Here's how the part is built. I have some questions about the finished solid (model axes, mm). Coordinates: 2 decimals unless noted, no trailing zeros. Write each loop counter-clockwise with the first axis right and the second up, starting at its lowest first coordinate (ties: lowest second). Pieces come first, ordered by that corner, then holes.
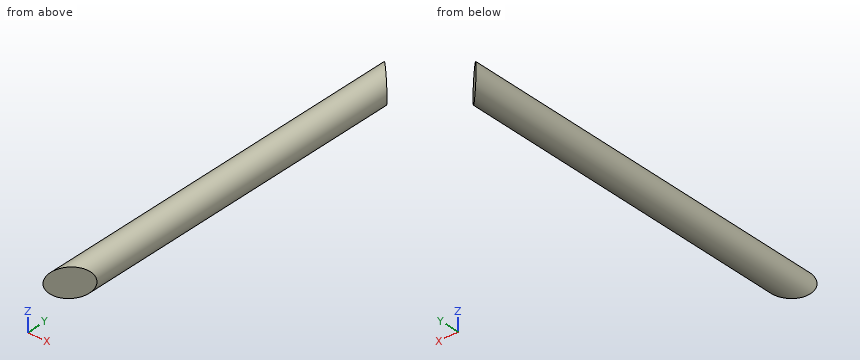
```python
from build123d import *

# Parameters (mm, degrees)
SKETCH1_R               = 31.75
BOSS_EXTRUDE1_DEPTH     = 723.9
SKETCH4_R               = 31.75
BOSS_EXTRUDE2_DEPTH     = 63.5
SKETCH5_R               = 31.75
BOSS_EXTRUDE3_DEPTH     = 63.5
CUT_EXTRUDE2_DEPTH      = 63.5
CUT_EXTRUDE2_DEPTH_BACK = 63.5


with BuildPart() as part:
    # Sketch1 → Boss-Extrude1 (new body)
    with BuildSketch(Plane(origin=(0, 0, 0), x_dir=(1, 0, 0), z_dir=(0, 1, 0))):
        Circle(SKETCH1_R)
    extrude(amount=BOSS_EXTRUDE1_DEPTH)

    # Sketch4 → Boss-Extrude2 (add)
    with BuildSketch(Plane(origin=(0, 723.9, 0), x_dir=(1, 0, 0), z_dir=(0, 1, 0))):
        Circle(SKETCH4_R)
    extrude(amount=BOSS_EXTRUDE2_DEPTH)

    # Sketch5 → Boss-Extrude3 (add)
    with BuildSketch(Plane.XZ):
        Circle(SKETCH5_R)
    extrude(amount=BOSS_EXTRUDE3_DEPTH)

    # Sketch2 → Cut-Extrude2 (cut, two sides)
    with BuildSketch(Plane.XY) as cut_extrude2_sk:
        Polygon((-31.75, -63.5), (31.75, -63.5), (31.75, 0), align=None)
        Polygon((31.75, 723.9), (-31.75, 787.4), (31.75, 787.4), align=None)
    extrude(amount=CUT_EXTRUDE2_DEPTH, mode=Mode.SUBTRACT)
    extrude(cut_extrude2_sk.sketch, amount=-CUT_EXTRUDE2_DEPTH_BACK, mode=Mode.SUBTRACT)


solid = part.part
```
1) Imagine slicing it at C-C on x = 0. Please give me the cut outline in (y, z).
Values follow:
outline: (-31.75, -31.75) - (755.65, -31.75) - (755.65, 31.75) - (-31.75, 31.75) - close
2) Imagine slicing it at B-B on y = 171. Please give me the cut outline in (x, z), then the cut area to 3 significant figures.
Values follow:
outline: circle Ø63.5 at (0, 0)
area: 3,170 mm2
3) I need wall thicknesses on probe 1 along X at (y, z) = (417.5, -2); probe 2 along Z at (x, y) = (3, 578.5); probe 3 along Y at (x, z) = (13, 9.5). Which ranges of each line are inside material? Lowest first, please.
Values follow:
probe 1: x = -31.69 to 31.69
probe 2: z = -31.61 to 31.61
probe 3: y = -18.75 to 742.65
4) Imagine slicing it at A-A on z = 0. Please give me the cut outline in (x, y).
Values follow:
outline: (-31.75, -63.5) - (31.75, 0) - (31.75, 723.9) - (-31.75, 787.4) - close
5) Will these pins go through, and if not, where does the flat tip stop? pin 1 (6 mm diameter, centred on x = -25, z = -14.5, fed in from +Y); pin 2 (4 mm diameter, centred on y = 378, z = -17, fed in from +X); pin 3 (1.5 mm diameter, centred on x = 12, y = 690, fed in from +Z).
Values follow:
pin 1: stops at y = 783.65
pin 2: stops at x = 27.98
pin 3: stops at z = 29.69
